Here's how the part is built. I have some questions about the finished solid (model axes, mm). Give positions to 0.01 mm unless a question says otherwise; leave off trailing zeros. Order: outer loops, then holes, each group sorted by start corner. A loop starts at its lowest first (then second) coordinate and runs counter-clockwise, first axis right, second up. Notation, with made-up numbers: M 12,67.5 L 30,67.5 A21 ccw 30,92.5 Z; hole C 48,68 d5. An arc over 180 degrees is marked long. Use one line per item in the form item = value.
from build123d import *

# Parameters (mm, degrees)
SZKIC1_W                        = 7
SZKIC1_H                        = 38
WYTNIJ_WYCI_GNI_CIE1_DEPTH      = 19
WYTNIJ_WYCI_GNI_CIE1_DEPTH_BACK = 19
SZKIC3_R                        = 14.5
WYTNIJ_WYCI_GNI_CIE2_DEPTH      = 8
WYTNIJ_WYCI_GNI_CIE2_DEPTH_BACK = 8
SFAZOWANIE1_SIZE                = 1.9


with BuildPart() as part:
    # Szkic1 → Obrót1 (revolve)
    with BuildSketch(Plane(origin=(0, 0, 0), x_dir=(1, 0, 0), z_dir=(0, 1, 0))):
        with BuildLine():
            Line((0, 18), (0, -22))
            Line((0, -22), (7, -22))
            Line((7, -22), (14.996070523, -9.955795743))
            ThreePointArc((14.996070523, -9.955795743), (15.861972188, 8.508691927), (0, 18))
        make_face()
        with Locations((3.5, -41)):
            Rectangle(SZKIC1_W, SZKIC1_H)
    revolve(axis=Axis((0, 0, -26.043516498), (0, 0, 1)))

    # Szkic2 → Wytnij-wyciągnięcie1 (cut, two sides)
    with BuildSketch(Plane(origin=(0, 0, 0), x_dir=(0, 0, -1), z_dir=(1, 0, 0))) as wytnij_wyci_gni_cie1_sk:
        with BuildLine():
            Line((-22, 7), (16.583123952, 7))
            ThreePointArc((16.583123952, 7), (5.192750307, 17.23471335), (-9.955795743, 14.996070523))
            Line((-9.955795743, 14.996070523), (-22, 7))
        make_face()
        with BuildLine():
            Line((-22, -7), (16.583123952, -7))
            ThreePointArc((16.583123952, -7), (5.192750307, -17.23471335), (-9.955795743, -14.996070523))
            Line((-9.955795743, -14.996070523), (-22, -7))
        make_face()
    extrude(amount=WYTNIJ_WYCI_GNI_CIE1_DEPTH, mode=Mode.SUBTRACT)
    extrude(wytnij_wyci_gni_cie1_sk.sketch, amount=-WYTNIJ_WYCI_GNI_CIE1_DEPTH_BACK, mode=Mode.SUBTRACT)

    # Szkic3 → Wytnij-wyciągnięcie2 (cut, two sides)
    with BuildSketch(Plane(origin=(0, 0, 0), x_dir=(1, 0, 0), z_dir=(0, 1, 0))) as wytnij_wyci_gni_cie2_sk:
        Circle(SZKIC3_R)
    extrude(amount=WYTNIJ_WYCI_GNI_CIE2_DEPTH, mode=Mode.SUBTRACT)
    extrude(wytnij_wyci_gni_cie2_sk.sketch, amount=-WYTNIJ_WYCI_GNI_CIE2_DEPTH_BACK, mode=Mode.SUBTRACT)

    # Sfazowanie1
    sfazowanie1_edges = [part.edges().sort_by_distance(p)[0] for p in [
        (-7, 0, 60),
    ]]
    chamfer(sfazowanie1_edges, length=SFAZOWANIE1_SIZE)


solid = part.part
Q1. Thinking about a two-plate mould opening in X: for faces 1 (the face through (-10.163, 0.224, 17.232)), 2 (the face through (6.691, 0.098, 12.864)), 3 (the face through (-3.8, -7, 14.2)), 4 (the face through (6.466, -2.681, 39.797)), which applies, +X half, -X half, draft (parallel to the pull), parting line (faces both ways), or undercut?
Found:
face_1 = -X half
face_2 = undercut
face_3 = draft
face_4 = parting line
Q2. I want a section at D-D on z = 13.5. Write out the boundary of the cut face in (x, y), then the cut area to 3 significant figures.
Found:
outline = M -10.53,-7 L -5.29,-7 L -5.29,7 L -10.53,7 A12.64 ccw Z; M 5.29,-7 L 10.53,-7 A12.64 ccw 10.53,7 L 5.29,7 Z
area = 187 mm²
Q3. I want a section at A-A on z = 0. Write out the boundary of the cut face in (x, y), then the cut area to 3 significant figures.
Found:
outline = M -16.58,-7 L -14.5,-7 L -14.5,7 L -16.58,7 A18 ccw Z; M 14.5,-7 L 16.58,-7 A18 ccw 16.58,7 L 14.5,7 Z
area = 85.0 mm²
Q4. I want a section at B-B on y = 0. Write out the boundary of the cut face in (x, z).
Found:
outline = M -15,9.96 A18 ccw long 15,9.96 L 7,22 L 7,58.1 L 5.1,60 L -5.1,60 L -7,58.1 L -7,22 Z; hole C 0,0 d29
Q5. I need wall thicknesses on L1, parallel to Z at x = 4, y = -5; L2, parallel to Z at x = 0, y = -3.5; L3, parallel to X at y = -1.5, z = 0. Which ranges of each line are inside material? Lowest first, please.
Found:
L1 = -16.82 to -13.94, 13.94 to 58.7
L2 = -17.66 to -14.5, 14.5 to 60
L3 = -17.94 to -14.5, 14.5 to 17.94
Q6. I want a section at C-C on z = 53. Write out the boundary of the cut face in (x, y), then the cut area to 3 significant figures.
Found:
outline = C 0,0 d14
area = 154 mm²
Q7. I'm going to push flat-ended pins straight in: pin 1 Ø2 at (y, z) = (1.5, 1) entering from -X; pin 2 Ø8 at (x, y) = (10, -3.5) entering from -Z; pin 3 Ø6 at (y, z) = (4.5, 49) entering from -X. Where does each tip first touch, or does it pass through?
Found:
pin_1 = -17.98
pin_2 = -16.75
pin_3 = -6.84
